from build123d import *

# Parameters (mm, degrees)
SKETCH1_W                   = 100
SKETCH1_H                   = 92
BOSS_EXTRUDE1_DEPTH         = 22.5
CHAMFER1_SIZE               = 5
SKETCH3_R                   = 7.5
BOSS_EXTRUDE2_DEPTH         = 1
M5_TAPPED_HOLE1_D           = 4.2
M5_TAPPED_HOLE1_DEPTH       = 5
M5_TAPPED_HOLE1_CSINK_D     = 5.05
M5_TAPPED_HOLE1_CSINK_ANGLE = 90
M5_TAPPED_HOLE1_TIP         = 1.2618073
SKETCH8_R                   = 2
BOSS_EXTRUDE3_DEPTH         = 15


with BuildPart() as part:
    # Sketch1 → Boss-Extrude1 (new body)
    with BuildSketch(Plane(origin=(0, 0, 0), x_dir=(1, 0, 0), z_dir=(0, 1, 0))):
        Rectangle(SKETCH1_W, SKETCH1_H)
    extrude(amount=BOSS_EXTRUDE1_DEPTH)

    # Chamfer1
    chamfer1_edges = [part.edges().sort_by_distance(p)[0] for p in [
        (50, 11.25, 46),
        (-50, 11.25, 46),
        (-50, 11.25, -46),
        (50, 11.25, -46),
    ]]
    chamfer(chamfer1_edges, length=CHAMFER1_SIZE)

    # Sketch3 → Boss-Extrude2 (add)
    with BuildSketch(Plane.XY.offset(46)):
        with Locations((-30, 11.25)):
            Circle(SKETCH3_R)
    extrude(amount=BOSS_EXTRUDE2_DEPTH)

    # M5 Tapped Hole1
    with Locations(Plane(origin=(0, 22.5, 0), x_dir=(1, 0, 0), z_dir=(0, 1, 0))):
        with Locations((-33, 40), (31, 40), (29, -40), (-16, -40)):
            CounterSinkHole(M5_TAPPED_HOLE1_D / 2, M5_TAPPED_HOLE1_CSINK_D / 2, depth=M5_TAPPED_HOLE1_DEPTH, counter_sink_angle=M5_TAPPED_HOLE1_CSINK_ANGLE)
            with Locations((0, 0, -(M5_TAPPED_HOLE1_DEPTH + M5_TAPPED_HOLE1_TIP / 2))):  # 118° drill point
                Cone(0, M5_TAPPED_HOLE1_D / 2, M5_TAPPED_HOLE1_TIP, mode=Mode.SUBTRACT)

    # Sketch8 → Boss-Extrude3 (add)
    with BuildSketch(Plane.ZY.offset(50)):
        with Locations((-29.407923946, 11.25)):
            Circle(SKETCH8_R)
        with Locations((-22.407923946, 11.25)):
            Circle(SKETCH8_R)
        with Locations((-15.407923946, 11.25)):
            Circle(SKETCH8_R)
    extrude(amount=BOSS_EXTRUDE3_DEPTH)


solid = part.part
The model under review builds one solid part; all positions refer to its coordinate system, in mm. A direction names the side the tool comes from. Coordinates: 2 decimals unless noted, no trailing zeros. Order: outer loops, then holes, each group sorted by start corner. A loop starts at its lowest first (then second) coordinate and runs counter-clockwise, first axis right, second up. Notation, with made-up numbers: (30, 38.5) -> (87, 38.5) arc R33 ccw to (87, 75.5) -> close; hole circle Ø4 at (-28, -27). An arc over 180 degrees is marked (long way). Answer in a Markdown table with one row per item.
(1) Machinability: for faces 1 (the flat face through (48, 11, 43)), 2 (the cylindrical face through (-57.395, 11.338, -17.406)), 3 (the cylindrical face through (31.46, 19.76, -37.95)), which of the approach directions +Z, -Z, +X, -X, +Y, -Y give a long, thin tool a straight path to every point of the face, cutting with its end or side? Answer none if there is none.
Answers:
| item | result |
|---|---|
| face 1 | +Z, +X, +Y, -Y |
| face 2 | -X |
| face 3 | +Y |
(2) Consider section B-B (z = 7.5). Write out the cut boundary in (x, y).
Answers:
| item | result |
|---|---|
| outline | (-50, 0) -> (50, 0) -> (50, 22.5) -> (-50, 22.5) -> close |
(3) Insertion check: pin 1 (1.5 mm diameter, centred on x = -38.5, y = 2.5, fed in from +Z); pin 2 (5 mm diameter, centred on x = -16, z = 40, fed in from +Y) (3 decimals); pin 3 (5 mm diameter, centred on y = 20, z = -13.5, fed in from -X). Each pin has a flat end and moves straight along its axis. Give the tip position at first contact, or say it passes through.
Answers:
| item | result |
|---|---|
| pin 1 | z = 46 |
| pin 2 | y = 22.475 |
| pin 3 | x = -50 |
(4) The part is to be moulded in two halves that separate along X. For faces 4 (the flat face through (-47, 11, -44)), 5 (the flat face through (-1, 22.5, -1)), 6 (the cylindrical face through (-31.334, 19.755, -38.722)), say which applies: +X half, -X half, draft (parallel to the pull), parting line (faces both ways), or undercut.
Answers:
| item | result |
|---|---|
| face 4 | -X half |
| face 5 | draft |
| face 6 | undercut |
(5) Wall thickness on line 1 along X through (y, z) = (20.5, 40); line 2 along X through (y, z) = (20.7, -40); line 3 along Z through (x, y) = (-16, 18.6): over which ranges is each line inside the solid? List them lowest first.
Answers:
| item | result |
|---|---|
| line 1 | -50 to -18.1, -13.9 to 26.9, 31.1 to 50 |
| line 2 | -50 to -35.1, -30.9 to 28.9, 33.1 to 50 |
| line 3 | -46 to 37.9, 42.1 to 46 |
(6) Consider section A-A (y = 11.25). Write out the cut boundary in (x, z).
Answers:
| item | result |
|---|---|
| outline | (-65, -31.41) -> (-50, -31.41) -> (-50, -41) -> (-45, -46) -> (45, -46) -> (50, -41) -> (50, 41) -> (45, 46) -> (-22.5, 46) -> (-22.5, 47) -> (-37.5, 47) -> (-37.5, 46) -> (-45, 46) -> (-50, 41) -> (-50, -13.41) -> (-65, -13.41) -> (-65, -17.41) -> (-50, -17.41) -> (-50, -20.41) -> (-65, -20.41) -> (-65, -24.41) -> (-50, -24.41) -> (-50, -27.41) -> (-65, -27.41) -> close |
